Design review of the part built by this model. Coordinates are the model's own, in mm. Coordinates: 2 decimals unless noted, no trailing zeros. Order: outer loops, then holes, each group sorted by start corner. A loop starts at its lowest first (then second) coordinate and runs counter-clockwise, first axis right, second up. Notation, with made-up numbers: M 74.25,33 L 129.25,33 A35 ccw 129.25,65 Z; hole C 1,-9.5 d5. An arc over 180 degrees is marked long. Answer as a JSON object with one key per item and string values.
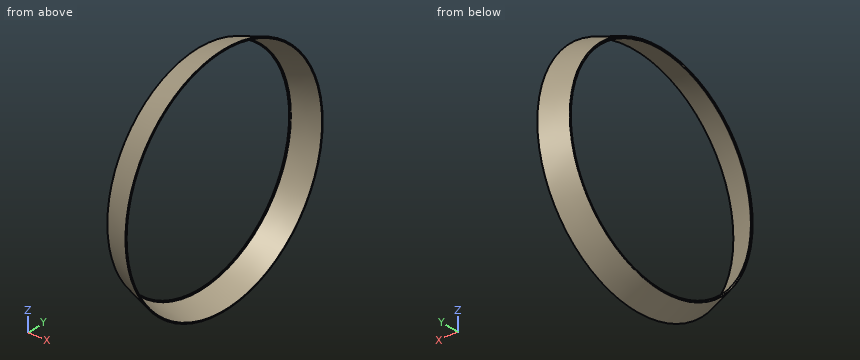
Autodesk Inventor part; units mm, degrees
ref_plane "cage_XY" through (0, 0, 0) normal (0, 0, 1) x (1, 0, 0)
ref_plane "cage_YZ" through (0, 0, 0) normal (1, 0, 0) x (0, 1, 0)
ref_plane "cage_ZX" through (0, 0, 0) normal (0, 1, 0) x (0, 0, 1)
sketch "Sketch_1" plane through (0, 0, 0) normal (0, 0, 1) x (1, 0, 0)
  line L0 (50, 0) -> (-50, 0)
  arc A0 (-0.1653, 102.1585) -> (-0.3576, 101.7856) centre (-0.0709, 101.8738) ccw
  line L1 (-0.3576, 101.7856) -> (-0.0028, 100.6321)
  line L2 (-0.0028, 100.6321) -> (0.9466, 100.947)
  line L3 (0.9466, 100.947) -> (0.8571, 101.238)
  arc A1 (0.9853, 101.4866) -> (0.8571, 101.238) centre (1.0482, 101.2968) ccw
  line L4 (0.9853, 101.4866) -> (24.0593, 109.1399)
  line L5 (24.0593, 109.1399) -> (23.7652, 110.096)
  line L6 (23.7652, 110.096) -> (-0.1653, 102.1585)
revolve "Revolution1" add sketch "Sketch_1" angle 360 about axis through (50, 0, 0) along (1, 0, 0)
ref_plane "cage_XY" through (0, 0, 0) normal (0, 0, 1) x (1, 0, 0)
ref_plane "cage_YZ" through (0, 0, 0) normal (1, 0, 0) x (0, 1, 0)
ref_plane "cage_ZX" through (0, 0, 0) normal (0, 1, 0) x (0, 0, 1)
ref_plane "roller1_XY" through (0, 100.0165, 0) normal (1, 0, 0) x (0, 0, -1)
ref_plane "roller1_YZ" through (0, 100.0165, 0) normal (0, 0, -1) x (0, 1, 0)
ref_plane "roller1_ZX" through (0, 100.0165, 0) normal (0, 1, 0) x (1, 0, 0)
ref_plane "roller10_XY" through (0, 4.2448, 99.9264) normal (1, 0, 0) x (0, 0.9991, -0.0424)
ref_plane "roller10_YZ" through (0, 4.2448, 99.9264) normal (0, 0.9991, -0.0424) x (0, 0.0424, 0.9991)
ref_plane "roller10_ZX" through (0, 4.2448, 99.9264) normal (0, 0.0424, 0.9991) x (1, 0, 0)
ref_plane "roller11_XY" through (0, -12.7039, 99.2064) normal (1, 0, 0) x (0, 0.9919, 0.127)
ref_plane "roller11_YZ" through (0, -12.7039, 99.2064) normal (0, 0.9919, 0.127) x (0, -0.127, 0.9919)
ref_plane "roller11_ZX" through (0, -12.7039, 99.2064) normal (0, -0.127, 0.9919) x (1, 0, 0)
ref_plane "roller12_XY" through (0, -29.2871, 95.6325) normal (1, 0, 0) x (0, 0.9562, 0.2928)
ref_plane "roller12_YZ" through (0, -29.2871, 95.6325) normal (0, 0.9562, 0.2928) x (0, -0.2928, 0.9562)
ref_plane "roller12_ZX" through (0, -29.2871, 95.6325) normal (0, -0.2928, 0.9562) x (1, 0, 0)
ref_plane "roller13_XY" through (0, -45.0278, 89.3073) normal (1, 0, 0) x (0, 0.8929, 0.4502)
ref_plane "roller13_YZ" through (0, -45.0278, 89.3073) normal (0, 0.8929, 0.4502) x (0, -0.4502, 0.8929)
ref_plane "roller13_ZX" through (0, -45.0278, 89.3073) normal (0, -0.4502, 0.8929) x (1, 0, 0)
ref_plane "roller14_XY" through (0, -59.4731, 80.413) normal (1, 0, 0) x (0, 0.804, 0.5946)
ref_plane "roller14_YZ" through (0, -59.4731, 80.413) normal (0, 0.804, 0.5946) x (0, -0.5946, 0.804)
ref_plane "roller14_ZX" through (0, -59.4731, 80.413) normal (0, -0.5946, 0.804) x (1, 0, 0)
ref_plane "roller15_XY" through (0, -72.2075, 69.2053) normal (1, 0, 0) x (0, 0.6919, 0.722)
ref_plane "roller15_YZ" through (0, -72.2075, 69.2053) normal (0, 0.6919, 0.722) x (0, -0.722, 0.6919)
ref_plane "roller15_ZX" through (0, -72.2075, 69.2053) normal (0, -0.722, 0.6919) x (1, 0, 0)
ref_plane "roller16_XY" through (0, -82.8646, 56.0067) normal (1, 0, 0) x (0, 0.56, 0.8285)
ref_plane "roller16_YZ" through (0, -82.8646, 56.0067) normal (0, 0.56, 0.8285) x (0, -0.8285, 0.56)
ref_plane "roller16_ZX" through (0, -82.8646, 56.0067) normal (0, -0.8285, 0.56) x (1, 0, 0)
ref_plane "roller17_XY" through (0, -91.1379, 41.1969) normal (1, 0, 0) x (0, 0.4119, 0.9112)
ref_plane "roller17_YZ" through (0, -91.1379, 41.1969) normal (0, 0.4119, 0.9112) x (0, -0.9112, 0.4119)
ref_plane "roller17_ZX" through (0, -91.1379, 41.1969) normal (0, -0.9112, 0.4119) x (1, 0, 0)
ref_plane "roller18_XY" through (0, -96.7893, 25.202) normal (1, 0, 0) x (0, 0.252, 0.9677)
ref_plane "roller18_YZ" through (0, -96.7893, 25.202) normal (0, 0.252, 0.9677) x (0, -0.9677, 0.252)
ref_plane "roller18_ZX" through (0, -96.7893, 25.202) normal (0, -0.9677, 0.252) x (1, 0, 0)
ref_plane "roller19_XY" through (0, -99.6562, 8.482) normal (1, 0, 0) x (0, 0.0848, 0.9964)
ref_plane "roller19_YZ" through (0, -99.6562, 8.482) normal (0, 0.0848, 0.9964) x (0, -0.9964, 0.0848)
ref_plane "roller19_ZX" through (0, -99.6562, 8.482) normal (0, -0.9964, 0.0848) x (1, 0, 0)
ref_plane "roller2_XY" through (0, 98.5779, 16.9029) normal (1, 0, 0) x (0, 0.169, -0.9856)
ref_plane "roller2_YZ" through (0, 98.5779, 16.9029) normal (0, 0.169, -0.9856) x (0, 0.9856, 0.169)
ref_plane "roller2_ZX" through (0, 98.5779, 16.9029) normal (0, 0.9856, 0.169) x (1, 0, 0)
ref_plane "roller20_XY" through (0, -99.6562, -8.482) normal (1, 0, 0) x (0, -0.0848, 0.9964)
ref_plane "roller20_YZ" through (0, -99.6562, -8.482) normal (0, -0.0848, 0.9964) x (0, -0.9964, -0.0848)
ref_plane "roller20_ZX" through (0, -99.6562, -8.482) normal (0, -0.9964, -0.0848) x (1, 0, 0)
ref_plane "roller21_XY" through (0, -96.7893, -25.202) normal (1, 0, 0) x (0, -0.252, 0.9677)
ref_plane "roller21_YZ" through (0, -96.7893, -25.202) normal (0, -0.252, 0.9677) x (0, -0.9677, -0.252)
ref_plane "roller21_ZX" through (0, -96.7893, -25.202) normal (0, -0.9677, -0.252) x (1, 0, 0)
ref_plane "roller22_XY" through (0, -91.1379, -41.1969) normal (1, 0, 0) x (0, -0.4119, 0.9112)
ref_plane "roller22_YZ" through (0, -91.1379, -41.1969) normal (0, -0.4119, 0.9112) x (0, -0.9112, -0.4119)
ref_plane "roller22_ZX" through (0, -91.1379, -41.1969) normal (0, -0.9112, -0.4119) x (1, 0, 0)
ref_plane "roller23_XY" through (0, -82.8646, -56.0067) normal (1, 0, 0) x (0, -0.56, 0.8285)
ref_plane "roller23_YZ" through (0, -82.8646, -56.0067) normal (0, -0.56, 0.8285) x (0, -0.8285, -0.56)
ref_plane "roller23_ZX" through (0, -82.8646, -56.0067) normal (0, -0.8285, -0.56) x (1, 0, 0)
ref_plane "roller24_XY" through (0, -72.2075, -69.2053) normal (1, 0, 0) x (0, -0.6919, 0.722)
ref_plane "roller24_YZ" through (0, -72.2075, -69.2053) normal (0, -0.6919, 0.722) x (0, -0.722, -0.6919)
ref_plane "roller24_ZX" through (0, -72.2075, -69.2053) normal (0, -0.722, -0.6919) x (1, 0, 0)
ref_plane "roller25_XY" through (0, -59.4731, -80.413) normal (1, 0, 0) x (0, -0.804, 0.5946)
ref_plane "roller25_YZ" through (0, -59.4731, -80.413) normal (0, -0.804, 0.5946) x (0, -0.5946, -0.804)
ref_plane "roller25_ZX" through (0, -59.4731, -80.413) normal (0, -0.5946, -0.804) x (1, 0, 0)
ref_plane "roller26_XY" through (0, -45.0278, -89.3073) normal (1, 0, 0) x (0, -0.8929, 0.4502)
ref_plane "roller26_YZ" through (0, -45.0278, -89.3073) normal (0, -0.8929, 0.4502) x (0, -0.4502, -0.8929)
ref_plane "roller26_ZX" through (0, -45.0278, -89.3073) normal (0, -0.4502, -0.8929) x (1, 0, 0)
ref_plane "roller27_XY" through (0, -29.2871, -95.6325) normal (1, 0, 0) x (0, -0.9562, 0.2928)
ref_plane "roller27_YZ" through (0, -29.2871, -95.6325) normal (0, -0.9562, 0.2928) x (0, -0.2928, -0.9562)
ref_plane "roller27_ZX" through (0, -29.2871, -95.6325) normal (0, -0.2928, -0.9562) x (1, 0, 0)
ref_plane "roller28_XY" through (0, -12.7039, -99.2064) normal (1, 0, 0) x (0, -0.9919, 0.127)
ref_plane "roller28_YZ" through (0, -12.7039, -99.2064) normal (0, -0.9919, 0.127) x (0, -0.127, -0.9919)
ref_plane "roller28_ZX" through (0, -12.7039, -99.2064) normal (0, -0.127, -0.9919) x (1, 0, 0)
ref_plane "roller29_XY" through (0, 4.2448, -99.9264) normal (1, 0, 0) x (0, -0.9991, -0.0424)
ref_plane "roller29_YZ" through (0, 4.2448, -99.9264) normal (0, -0.9991, -0.0424) x (0, 0.0424, -0.9991)
ref_plane "roller29_ZX" through (0, 4.2448, -99.9264) normal (0, 0.0424, -0.9991) x (1, 0, 0)
ref_plane "roller3_XY" through (0, 94.3033, 33.3195) normal (1, 0, 0) x (0, 0.3331, -0.9429)
ref_plane "roller3_YZ" through (0, 94.3033, 33.3195) normal (0, 0.3331, -0.9429) x (0, 0.9429, 0.3331)
ref_plane "roller3_ZX" through (0, 94.3033, 33.3195) normal (0, 0.9429, 0.3331) x (1, 0, 0)
ref_plane "roller30_XY" through (0, 21.0714, -97.7717) normal (1, 0, 0) x (0, -0.9776, -0.2107)
ref_plane "roller30_YZ" through (0, 21.0714, -97.7717) normal (0, -0.9776, -0.2107) x (0, 0.2107, -0.9776)
ref_plane "roller30_ZX" through (0, 21.0714, -97.7717) normal (0, 0.2107, -0.9776) x (1, 0, 0)
ref_plane "roller31_XY" through (0, 37.2918, -92.8042) normal (1, 0, 0) x (0, -0.9279, -0.3729)
ref_plane "roller31_YZ" through (0, 37.2918, -92.8042) normal (0, -0.9279, -0.3729) x (0, 0.3729, -0.9279)
ref_plane "roller31_ZX" through (0, 37.2918, -92.8042) normal (0, 0.3729, -0.9279) x (1, 0, 0)
ref_plane "roller32_XY" through (0, 52.4394, -85.167) normal (1, 0, 0) x (0, -0.8515, -0.5243)
ref_plane "roller32_YZ" through (0, 52.4394, -85.167) normal (0, -0.8515, -0.5243) x (0, 0.5243, -0.8515)
ref_plane "roller32_ZX" through (0, 52.4394, -85.167) normal (0, 0.5243, -0.8515) x (1, 0, 0)
ref_plane "roller33_XY" through (0, 66.0784, -75.0796) normal (1, 0, 0) x (0, -0.7507, -0.6607)
ref_plane "roller33_YZ" through (0, 66.0784, -75.0796) normal (0, -0.7507, -0.6607) x (0, 0.6607, -0.7507)
ref_plane "roller33_ZX" through (0, 66.0784, -75.0796) normal (0, 0.6607, -0.7507) x (1, 0, 0)
ref_plane "roller34_XY" through (0, 77.8164, -62.8324) normal (1, 0, 0) x (0, -0.6282, -0.778)
ref_plane "roller34_YZ" through (0, 77.8164, -62.8324) normal (0, -0.6282, -0.778) x (0, 0.778, -0.6282)
ref_plane "roller34_ZX" through (0, 77.8164, -62.8324) normal (0, 0.778, -0.6282) x (1, 0, 0)
ref_plane "roller35_XY" through (0, 87.3158, -48.7775) normal (1, 0, 0) x (0, -0.4877, -0.873)
ref_plane "roller35_YZ" through (0, 87.3158, -48.7775) normal (0, -0.4877, -0.873) x (0, 0.873, -0.4877)
ref_plane "roller35_ZX" through (0, 87.3158, -48.7775) normal (0, 0.873, -0.4877) x (1, 0, 0)
ref_plane "roller36_XY" through (0, 94.3033, -33.3195) normal (1, 0, 0) x (0, -0.3331, -0.9429)
ref_plane "roller36_YZ" through (0, 94.3033, -33.3195) normal (0, -0.3331, -0.9429) x (0, 0.9429, -0.3331)
ref_plane "roller36_ZX" through (0, 94.3033, -33.3195) normal (0, 0.9429, -0.3331) x (1, 0, 0)
ref_plane "roller37_XY" through (0, 98.5779, -16.9029) normal (1, 0, 0) x (0, -0.169, -0.9856)
ref_plane "roller37_YZ" through (0, 98.5779, -16.9029) normal (0, -0.169, -0.9856) x (0, 0.9856, -0.169)
ref_plane "roller37_ZX" through (0, 98.5779, -16.9029) normal (0, 0.9856, -0.169) x (1, 0, 0)
ref_plane "roller4_XY" through (0, 87.3158, 48.7775) normal (1, 0, 0) x (0, 0.4877, -0.873)
ref_plane "roller4_YZ" through (0, 87.3158, 48.7775) normal (0, 0.4877, -0.873) x (0, 0.873, 0.4877)
ref_plane "roller4_ZX" through (0, 87.3158, 48.7775) normal (0, 0.873, 0.4877) x (1, 0, 0)
ref_plane "roller5_XY" through (0, 77.8164, 62.8324) normal (1, 0, 0) x (0, 0.6282, -0.778)
ref_plane "roller5_YZ" through (0, 77.8164, 62.8324) normal (0, 0.6282, -0.778) x (0, 0.778, 0.6282)
ref_plane "roller5_ZX" through (0, 77.8164, 62.8324) normal (0, 0.778, 0.6282) x (1, 0, 0)
ref_plane "roller6_XY" through (0, 66.0784, 75.0796) normal (1, 0, 0) x (0, 0.7507, -0.6607)
ref_plane "roller6_YZ" through (0, 66.0784, 75.0796) normal (0, 0.7507, -0.6607) x (0, 0.6607, 0.7507)
ref_plane "roller6_ZX" through (0, 66.0784, 75.0796) normal (0, 0.6607, 0.7507) x (1, 0, 0)
ref_plane "roller7_XY" through (0, 52.4394, 85.167) normal (1, 0, 0) x (0, 0.8515, -0.5243)
ref_plane "roller7_YZ" through (0, 52.4394, 85.167) normal (0, 0.8515, -0.5243) x (0, 0.5243, 0.8515)
ref_plane "roller7_ZX" through (0, 52.4394, 85.167) normal (0, 0.5243, 0.8515) x (1, 0, 0)
ref_plane "roller8_XY" through (0, 37.2918, 92.8042) normal (1, 0, 0) x (0, 0.9279, -0.3729)
ref_plane "roller8_YZ" through (0, 37.2918, 92.8042) normal (0, 0.9279, -0.3729) x (0, 0.3729, 0.9279)
ref_plane "roller8_ZX" through (0, 37.2918, 92.8042) normal (0, 0.3729, 0.9279) x (1, 0, 0)
ref_plane "roller9_XY" through (0, 21.0714, 97.7717) normal (1, 0, 0) x (0, 0.9776, -0.2107)
ref_plane "roller9_YZ" through (0, 21.0714, 97.7717) normal (0, 0.9776, -0.2107) x (0, 0.2107, 0.9776)
ref_plane "roller9_ZX" through (0, 21.0714, 97.7717) normal (0, 0.2107, 0.9776) x (1, 0, 0)
properties part number "T4DB 170_cage"
1) Insertion check: pin 1 Ø1.5 at (x, z) = (13.5, -34.5) entering from +Y; pin 2 Ø1.5 at (x, y) = (10, 63.5) entering from +Z; pin 3 Ø10 at (x, y) = (10.5, 32.5) entering from +Z. Each pin has a flat end and moves straight along its axis. Give the tip position at first contact, or say it passes through.
Taken from the geometry:
{"pin 1": "stops at y = 101.32", "pin 2": "stops at z = 84.93", "pin 3": "stops at z = 102.88"}
2) To check wall thickness, follow L1, parallel to Z at x = 6, y = -80.5; L2, parallel to Z at x = 7.5, y = 75.5; L3, parallel to Y at x = 22.75, z = -20. State the ranges of each line that lie inside material, in increasing order.
Taken from the geometry:
{"L1": "z = -66.17 to -64.5, 64.5 to 66.17", "L2": "z = -72.54 to -71.01, 71.01 to 72.54", "L3": "y = -107.92 to -106.85, 106.85 to 107.92"}
3) Add section C-C (x = 19.5). State the section outline as (y, z) points, and give its area (3 significant figures).
Taken from the geometry:
{"outline": "C 0,0 d217.36; hole C 0,0 d215.26", "area": "716 mm2"}
4) Add section A-A (z = 0). State the section outline as (x, y) points.
Taken from the geometry:
{"outline": "M -0.36,-101.79 A0.3 ccw -0.17,-102.16 L 23.77,-110.1 L 24.06,-109.14 L 0.99,-101.49 A0.2 cw 0.86,-101.24 L 0.95,-100.95 L 0,-100.63 Z; M -0.36,101.79 L 0,100.63 L 0.95,100.95 L 0.86,101.24 A0.2 cw 0.99,101.49 L 24.06,109.14 L 23.77,110.1 L -0.17,102.16 A0.3 ccw Z"}
